from build123d import *

# Parameters (mm, degrees)
SKETCH1_R               = 4.3
SKETCH1_W               = 12.5
SKETCH1_H               = 12.5
BOSS_EXTRUDE1_DEPTH     = 8
CUT_EXTRUDE1_DEPTH      = 8
SKETCH1_2_R             = 4.3
SKETCH1_2_W             = 12.5
SKETCH1_2_H             = 12.5
BOSS_EXTRUDE2_DEPTH     = 10
CUT_EXTRUDE2_DEPTH      = 3
CUT_EXTRUDE2_DEPTH_BACK = 9
SKETCH3_W               = 12.5
SKETCH3_H               = 12.5
BOSS_EXTRUDE3_DEPTH     = 2
SKETCH4_R               = 4.3
BOSS_EXTRUDE5_DEPTH     = 2
BOSS_EXTRUDE6_DEPTH     = 10
BOSS_EXTRUDE7_DEPTH     = 10
BOSS_EXTRUDE8_DEPTH     = 10


with BuildPart() as part:
    # Sketch1 → Boss-Extrude1 (new body)
    with BuildSketch(Plane.XY):
        with BuildLine():
            Line((-85.345346062, -25.7), (87.254653938, -25.7))
            Line((87.254653938, -25.7), (87.254653938, 0))
            ThreePointArc((87.254653938, 0), (85.409426659, 4.454772721), (80.954653938, 6.3))
            Line((80.954653938, 6.3), (-79.045346062, 6.3))
            ThreePointArc((-79.045346062, 6.3), (-83.500118784, 4.454772721), (-85.345346062, 0))
            Line((-85.345346062, 0), (-85.345346062, -25.7))
        make_face()
        with Locations((-79.045346062, 0)):
            Circle(SKETCH1_R, mode=Mode.SUBTRACT)
        with Locations((80.954653938, 0)):
            Circle(SKETCH1_R, mode=Mode.SUBTRACT)
        with Locations((-77.095346062, -17.45)):
            Rectangle(SKETCH1_W, SKETCH1_H, mode=Mode.SUBTRACT)
        with Locations((79.004653938, -17.45)):
            Rectangle(SKETCH1_W, SKETCH1_H, mode=Mode.SUBTRACT)
    extrude(amount=BOSS_EXTRUDE1_DEPTH)

    # Sketch2 → Cut-Extrude1 (cut)
    with BuildSketch(Plane.XY.offset(8)):
        with BuildLine():
            Line((-35.345346062, 3.5), (37.254653938, 3.5))
            ThreePointArc((37.254653938, 3.5), (40.754653938, 0), (37.254653938, -3.5))
            Line((37.254653938, -3.5), (-35.345346062, -3.5))
            ThreePointArc((-35.345346062, -3.5), (-38.845346062, 0), (-35.345346062, 3.5))
        make_face()
        with BuildLine():
            Line((-35.345346062, -13.95), (37.254653938, -13.95))
            ThreePointArc((37.254653938, -13.95), (40.754653938, -17.45), (37.254653938, -20.95))
            Line((37.254653938, -20.95), (34.643207431, -20.95))
            Line((34.643207431, -20.95), (-35.345346062, -20.95))
            ThreePointArc((-35.345346062, -20.95), (-38.845346062, -17.45), (-35.345346062, -13.95))
        make_face()
    extrude(amount=-CUT_EXTRUDE1_DEPTH, mode=Mode.SUBTRACT)

    # Sketch1<2> → Boss-Extrude2 (add)
    with BuildSketch(Plane.XY):
        with BuildLine():
            Line((-85.345346062, -25.7), (87.254653938, -25.7))
            Line((87.254653938, -25.7), (87.254653938, 0))
            ThreePointArc((87.254653938, 0), (85.409426659, 4.454772721), (80.954653938, 6.3))
            Line((80.954653938, 6.3), (-79.045346062, 6.3))
            ThreePointArc((-79.045346062, 6.3), (-83.500118784, 4.454772721), (-85.345346062, 0))
            Line((-85.345346062, 0), (-85.345346062, -25.7))
        make_face()
        with Locations((-79.045346062, 0)):
            Circle(SKETCH1_2_R, mode=Mode.SUBTRACT)
        with Locations((80.954653938, 0)):
            Circle(SKETCH1_2_R, mode=Mode.SUBTRACT)
        with Locations((-77.095346062, -17.45)):
            Rectangle(SKETCH1_2_W, SKETCH1_2_H, mode=Mode.SUBTRACT)
        with Locations((79.004653938, -17.45)):
            Rectangle(SKETCH1_2_W, SKETCH1_2_H, mode=Mode.SUBTRACT)
    extrude(amount=BOSS_EXTRUDE2_DEPTH)

    # Sketch2<2> → Cut-Extrude2 (cut, two sides)
    with BuildSketch(Plane.XY.offset(8)) as cut_extrude2_sk:
        with BuildLine():
            Line((-35.345346062, 3.5), (37.254653938, 3.5))
            ThreePointArc((37.254653938, 3.5), (40.754653938, 0), (37.254653938, -3.5))
            Line((37.254653938, -3.5), (-35.345346062, -3.5))
            ThreePointArc((-35.345346062, -3.5), (-38.845346062, 0), (-35.345346062, 3.5))
        make_face()
        with BuildLine():
            Line((-35.345346062, -13.95), (37.254653938, -13.95))
            ThreePointArc((37.254653938, -13.95), (40.754653938, -17.45), (37.254653938, -20.95))
            Line((37.254653938, -20.95), (34.643207431, -20.95))
            Line((34.643207431, -20.95), (-35.345346062, -20.95))
            ThreePointArc((-35.345346062, -20.95), (-38.845346062, -17.45), (-35.345346062, -13.95))
        make_face()
    extrude(amount=CUT_EXTRUDE2_DEPTH, mode=Mode.SUBTRACT)
    extrude(cut_extrude2_sk.sketch, amount=-CUT_EXTRUDE2_DEPTH_BACK, mode=Mode.SUBTRACT)

    # Sketch3 → Boss-Extrude3 (add)
    with BuildSketch(Plane.XY.offset(10)):
        with Locations((-77.095346062, -17.45)):
            Rectangle(SKETCH3_W, SKETCH3_H)
        with Locations((79.004653938, -17.45)):
            Rectangle(SKETCH3_W, SKETCH3_H)
    extrude(amount=-BOSS_EXTRUDE3_DEPTH)

    # Sketch4 → Boss-Extrude5 (add)
    with BuildSketch(Plane.XY.offset(10)):
        with Locations((-79.045346062, 0)):
            Circle(SKETCH4_R)
        with Locations((80.954653938, 0)):
            Circle(SKETCH4_R)
    extrude(amount=-BOSS_EXTRUDE5_DEPTH)

    # Sketch5 → Boss-Extrude6 (add)
    with BuildSketch(Plane.XY.offset(10)):
        with BuildLine():
            Line((-4.545346062, 3.5), (6.454653938, 3.5))
            ThreePointArc((6.454653938, 3.5), (2.954653938, 0), (6.454653938, -3.5))
            Line((6.454653938, -3.5), (-4.545346062, -3.5))
            ThreePointArc((-4.545346062, -3.5), (-1.045346062, 0), (-4.545346062, 3.5))
        make_face()
    extrude(amount=-BOSS_EXTRUDE6_DEPTH)

    # Sketch6 → Boss-Extrude7 (add)
    with BuildSketch(Plane.XY.offset(10)):
        with BuildLine():
            Line((-4.545346062, -13.95), (6.454653938, -13.95))
            ThreePointArc((6.454653938, -13.95), (2.954653938, -17.45), (6.454653938, -20.95))
            Line((6.454653938, -20.95), (-4.545346062, -20.95))
            ThreePointArc((-4.545346062, -20.95), (-1.045346062, -17.45), (-4.545346062, -13.95))
        make_face()
    extrude(amount=-BOSS_EXTRUDE7_DEPTH)

    # Sketch7 → Boss-Extrude8 (add)
    with BuildSketch(Plane.XY.offset(10)):
        with BuildLine():
            Line((-85.345346062, -25.7), (-85.345346062, -36.7))
            Line((-85.345346062, -36.7), (-65.345346062, -36.7))
            ThreePointArc((-65.345346062, -36.7), (-62.123520655, -28.921825407), (-54.345346062, -25.7))
            Line((-54.345346062, -25.7), (-85.345346062, -25.7))
        make_face()
        with BuildLine():
            Line((87.254653938, -25.7), (87.254653938, -36.7))
            Line((87.254653938, -36.7), (67.254653938, -36.7))
            ThreePointArc((67.254653938, -36.7), (64.032828531, -28.921825407), (56.254653938, -25.7))
            Line((56.254653938, -25.7), (87.254653938, -25.7))
        make_face()
    extrude(amount=-BOSS_EXTRUDE8_DEPTH)


solid = part.part
The listing builds one solid part. Answer for the finished solid, in the listing's coordinates (mm). A direction names the side the tool comes from. Give positions to 0.01 mm unless a question says otherwise; leave off trailing zeros. Write each loop counter-clockwise with the first axis right and the second up, starting at its lowest first coordinate (ties: lowest second). Pieces come first, ordered by that corner, then holes.
1) Section C-C (y = -2) is taken. Write down the section's boundary in (x, z).
2) Find the intervals of material crossed by L1, parallel to X at y = -12, z = 0.75; L2, parallel to Y at x = -19, z = 7.5; L3, parallel to Y at x = -37.5, z = 4.5, in increasing order.
3) Section A-A (y = -17.45) is taken. Write down the section's boundary in (x, z).
4) Section B-B (z = 3) is taken. Count the separate pieces of the cut face and the enclosed holes in it, and give its area (3 significant figures).
5) A tool of negligible diameter and unlimited length cuts with its end or side. For faces 5 (the face through (-38.844, -0.077, 4.93)), 6 (the face through (0, -25.7, 5)), 7 (the face through (-77, -23.7, 4)), from which of +Z, -Z, +X, -X, +Y, -Y can it reach the whole face along a straight path? Write none if from no direction.
6) For a pull along Y with two mould halves and no side action, classify faces 1 (the face through (22, -13.95, 5)), 2 (the face through (2.956, -17.373, 5.07)), 3 (the face through (0, -10, 10)), 4 (the face through (2, 6.3, 5)) as pulls with the +Y half, pulls with the -Y half, needs draft (parallel to the pull), parting line crosses it, or undercut.
7) Given P1, Ø6, axis at x = -33.5, z = 4, coming from the -Y side; P2, Ø6, axis at x = -77.5, y = -15, coming from the -Z side, each flat-ended and moving along its own axis, determine where each tip first touches the part or whether it passes through.
Response:
1. outline: (-85.35, 0) - (-82.85, 0) - (-82.85, 8) - (-75.24, 8) - (-75.24, 0) - (-38.22, 0) - (-38.22, 10) - (-85.35, 10) - close; (-1.67, 0) - (3.58, 0) - (3.58, 10) - (-1.67, 10) - close; (40.13, 0) - (77.15, 0) - (77.15, 8) - (84.76, 8) - (84.76, 0) - (87.25, 0) - (87.25, 10) - (40.13, 10) - close
2. L1: x = -85.35 to -83.35, -70.85 to 72.75, 85.25 to 87.25
2. L2: y = -25.7 to -20.95, -13.95 to -3.5, 3.5 to 6.3
2. L3: y = -25.7 to -20.21, -14.69 to -2.76, 2.76 to 6.3
3. outline: (-85.35, 0) - (-83.35, 0) - (-83.35, 8) - (-70.85, 8) - (-70.85, 0) - (-38.85, 0) - (-38.85, 10) - (-85.35, 10) - close; (-1.05, 0) - (2.95, 0) - (2.95, 10) - (-1.05, 10) - close; (40.75, 0) - (72.75, 0) - (72.75, 8) - (85.25, 8) - (85.25, 0) - (87.25, 0) - (87.25, 10) - (40.75, 10) - close
4. separate pieces: 1
4. enclosed holes: 8
4. area: 4,550 mm2
5. face 5: +Z, -Z
5. face 6: +Z, -Z, -Y
5. face 7: -Z
6. face 1: undercut
6. face 2: undercut
6. face 3: needs draft
6. face 4: pulls with the +Y half
7. P1: stops at y = -25.7
7. P2: stops at z = 8
